from build123d import *

# Parameters (mm, degrees)
F0_W     = 100
F0_H     = 70
F1_DEPTH = 6
F2_R     = 2
F3_W     = 10
F3_H     = 60
F4_DEPTH = 2


with BuildPart() as f1:
    # F0 (on Top) → F1 (new body)
    with BuildSketch(Plane.XY):
        Rectangle(F0_W, F0_H)
    extrude(amount=F1_DEPTH)

    # F2
    f2_edges = [f1.edges().sort_by_distance(p)[0] for p in [
        (0, -35, 0),
        (50, 0, 0),
        (0, 35, 0),
        (-50, 0, 0),
    ]]
    fillet(f2_edges, radius=F2_R)

    # F3 (on face) → F4 (cut)
    with BuildSketch(Plane.XY.offset(6)):
        with Locations((-40, 0)):
            Rectangle(F3_W, F3_H)
    extrude(amount=-F4_DEPTH, mode=Mode.SUBTRACT)


solid = f1.part
Build history of the part. All positions in model axes, mm. A direction names the side the tool comes from. Give positions to 0.01 mm unless a question says otherwise; leave off trailing zeros. Order: outer loops, then holes, each group sorted by start corner. A loop starts at its lowest first (then second) coordinate and runs counter-clockwise, first axis right, second up. Notation, with made-up numbers: M -27.5,2.5 L 16.5,2.5 A21 cw 16.5,18.5 Z; hole C 2,-39.75 d7. An arc over 180 degrees is marked long. Use one line per item in the form item = value.
Q1. Which spindle directions (+Z, -Z, +X, -X, +Y, -Y) get a long thin tool onto all of the face, cutting with end or side? Do faces 5 (the flat face through (-1, 35, 4)), 6 (the flat face through (-35, 0, 5)). Say none if no direction does.
Conclusion:
face_5 = +Z, -Z, +X, -X, +Y
face_6 = +Z
Q2. Pin check, flat tips, straight feed: P1, Ø5, axis at x = -41, y = 1, coming from the +Z side; P2, Ø1.5, axis at y = -13, z = 1, coming from the -X side. Stop position of each tip, or through.
Conclusion:
P1 = 4
P2 = -49.98
Q3. Wall check: probe 1 along Y at (x, z) = (-43, 5.2); probe 2 along X at (y, z) = (6, 4.1); probe 3 along Y at (x, z) = (-27.5, 1.7). Give the ranges that are in metal, low to high.
Conclusion:
probe_1 = -35 to -30, 30 to 35
probe_2 = -50 to -45, -35 to 50
probe_3 = -34.98 to 34.98
Q4. Slice it at B-B, the plane y = 1. Write the cut outline in (x, z).
Conclusion:
outline = M -50,2 A2 ccw -48,0 L 48,0 A2 ccw 50,2 L 50,6 L -35,6 L -35,4 L -45,4 L -45,6 L -50,6 Z
Q5. Pull direction X, two halves, no side cores. Call faces 1 (the flat face through (-50, 0, 4)), 2 (the flat face through (50, 0, 4)), 3 (the flat face through (-40, -30, 5)), 4 (the flat face through (-40, 0, 4)): released by +X, released by -X, zero draft, split by the parting line, or undercut.
Conclusion:
face_1 = released by -X
face_2 = released by +X
face_3 = undercut
face_4 = undercut
Q6. Slice it at A-A, the plane z = 5. Write the cut outline in (x, y).
Conclusion:
outline = M -50,-35 L 50,-35 L 50,35 L -50,35 Z; hole M -45,-30 L -35,-30 L -35,30 L -45,30 Z
